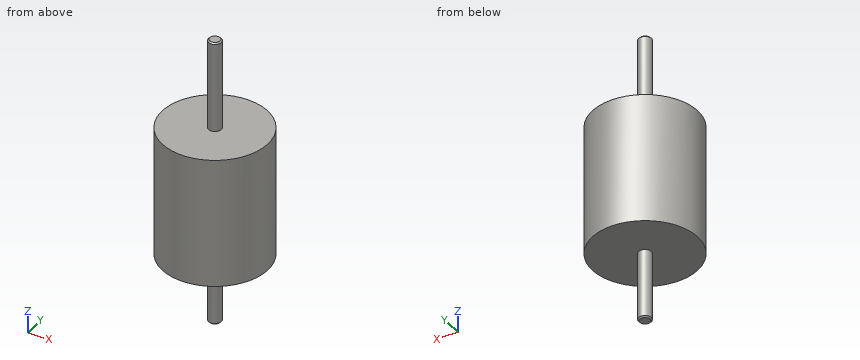
from build123d import *

# Parameters (mm, degrees)
SKETCH1_R           = 1.5
BOSS_EXTRUDE1_DEPTH = 33.5
SKETCH2_R           = 12.25
SKETCH2_R_2         = 1.5
BOSS_EXTRUDE2_DEPTH = 30
CHAMFER1_SIZE       = 0.3


with BuildPart() as part:
    # Sketch1 → Boss-Extrude1 (new body, symmetric)
    with BuildSketch(Plane.XY):
        Circle(SKETCH1_R)
    extrude(amount=BOSS_EXTRUDE1_DEPTH, both=True)

    # Sketch2 → Boss-Extrude2 (add)
    with BuildSketch(Plane.XY.offset(12.5)):
        Circle(SKETCH2_R)
        Circle(SKETCH2_R_2, mode=Mode.SUBTRACT)
    extrude(amount=-BOSS_EXTRUDE2_DEPTH)

    # Chamfer1
    chamfer1_edges = [part.edges().sort_by_distance(p)[0] for p in [
        (-1.5, 0, -33.5),
        (-1.5, 0, 33.5),
    ]]
    chamfer(chamfer1_edges, length=CHAMFER1_SIZE)


solid = part.part
For this review, take the finished solid that the model builds, in its own axes (mm). Round coordinates to 2 decimals unless told otherwise and drop trailing zeros. Write each loop counter-clockwise with the first axis right and the second up, starting at its lowest first coordinate (ties: lowest second). Pieces come first, ordered by that corner, then holes. Notation, with made-up numbers: M 88.5,13 L 146.5,13 A21 ccw 146.5,43 Z; hole C 34.25,62 d9. An arc over 180 degrees is marked long. Write item = value, one per line. Start each with the question number.
(1) We need section C-C (z = 5.5). Give the boundary of the cut face in (x, y).
(2) We need section D-D (z = -20.5). Give the boundary of the cut face in (x, y), then the cut area to 3 significant figures.
(3) Clearance check with flat-ended pins moving along their axes: pin 1 Ø10 at (y, z) = (-8, -12) entering from -X; pin 2 Ø4 at (y, z) = (4.5, 0) entering from +X; pin 3 Ø4 at (x, y) = (4, 9.5) entering from -Z; pin 4 Ø8 at (x, z) = (7.5, 18.5) entering from -Y (3 decimals). State where each tip first meets the part, or that it passes through.
(4) For line 1 along Z through (x, y) = (-10, -5.75); line 2 along X through (y, z) = (2.5, -4); line 3 along X through (y, z) = (-2.75, 3.5), list the stretches that pass through material, from the lowest coordinate up.
(5) We need section A-A (y = 0). Give the boundary of the cut face in (x, z).
Results found:
q1.outline = C 0,0 d24.5
q2.outline = C 0,0 d3
q2.area = 7.07 mm²
q3.pin_1 = -11.88
q3.pin_2 = 11.99
q3.pin_3 = -17.5
q3.pin_4 = through
q4.line_1 = -17.5 to 12.5
q4.line_2 = -11.99 to 11.99
q4.line_3 = -11.94 to 11.94
q5.outline = M -12.25,-17.5 L -1.5,-17.5 L -1.5,-33.2 L -1.2,-33.5 L 1.2,-33.5 L 1.5,-33.2 L 1.5,-17.5 L 12.25,-17.5 L 12.25,12.5 L 1.5,12.5 L 1.5,33.2 L 1.2,33.5 L -1.2,33.5 L -1.5,33.2 L -1.5,12.5 L -12.25,12.5 Z
